Model file for the job. Use its own axes, mm. Give positions to 0.01 mm unless a question says otherwise; leave off trailing zeros. Loops run counter-clockwise (first coordinate to the right, second up) from the corner with the lowest first, then second, coordinate; pieces in that order, holes last. Notation, with made-up numbers: M 83,-15 L 111,-15 A13 ccw 111,8 Z; hole C -8.75,58 d5. An arc over 180 degrees is marked long. Answer in a Markdown table with one row per item.
```python
from build123d import *
from OCP.BRepFilletAPI import BRepFilletAPI_MakeChamfer

# Parameters (mm, degrees)
BOSS_EXTRUDE1_DEPTH = 3
SKETCH2_R           = 2.5
BOSS_EXTRUDE2_DEPTH = 19
LPATTERN1_COUNT     = 2
LPATTERN1_PITCH     = 40
CHAMFER3_SIZE       = 1
CHAMFER3_SIZE2      = 0.624869352
FILLET1_R           = 10
SKETCH_1_R          = 2
CUT_EXTRUDE_1_DEPTH = 49.039445083


with BuildPart() as part:
    # Sketch1 → Boss-Extrude1 (new body)
    with BuildSketch(Plane(origin=(0, 0, 0), x_dir=(1, 0, 0), z_dir=(0, 1, 0))):
        with BuildLine():
            Line((-35, 17.5), (35, 17.5))
            ThreePointArc((35, 17.5), (38.535533906, 16.035533906), (40, 12.5))
            Line((40, 12.5), (40, -17.5))
            Line((40, -17.5), (-40, -17.5))
            Line((-40, -17.5), (-40, 12.5))
            ThreePointArc((-40, 12.5), (-38.535533906, 16.035533906), (-35, 17.5))
        make_face()
    extrude(amount=BOSS_EXTRUDE1_DEPTH)

    # Sketch2 → Boss-Extrude2 (add)
    with BuildSketch(Plane(origin=(40, 0, 0), x_dir=(0, 0, -1), z_dir=(1, 0, 0))):
        with BuildLine():
            Line((-21.372983346, 0), (-17.5, 0))
            Line((-17.5, 0), (-17.5, 3))
            ThreePointArc((-17.5, 3), (-23.822473089, 7.16227766), (-21.372983346, 0))
        make_face()
        with Locations((-21.372983346, 4)):
            Circle(SKETCH2_R, mode=Mode.SUBTRACT)
    boss_extrude2 = extrude(amount=-BOSS_EXTRUDE2_DEPTH)

    # LPattern1: Boss-Extrude2 ×2
    with Locations(*[(-i * LPATTERN1_PITCH, 0, 0) for i in range(1, LPATTERN1_COUNT)]):
        add(boss_extrude2)

    # Chamfer3: one chamfer whose edges measure the first distance from different faces: ONE call of the kernel's chamfer builder (chamfer() names one face for all edges)
    chamfer3_edges_1 = [part.edges().sort_by_distance(p)[0] for p in [
        (-29.5, 3, 17.5),
    ]]
    chamfer3_side_1 = [part.faces().sort_by_distance(p)[0] for p in [
        (-29.5, 1.5, 17.5),
    ]]
    chamfer3_edges_2 = [part.edges().sort_by_distance(p)[0] for p in [
        (10.5, 3, 17.5),
    ]]
    chamfer3_side_2 = [part.faces().sort_by_distance(p)[0] for p in [
        (10.5, 1.5, 17.5),
    ]]
    chamfer3 = BRepFilletAPI_MakeChamfer(part.part.solid().wrapped)
    for e in chamfer3_edges_1:
        chamfer3.Add(CHAMFER3_SIZE, CHAMFER3_SIZE2, e.wrapped, chamfer3_side_1[0].wrapped)  # the first distance lies on this face
    for e in chamfer3_edges_2:
        chamfer3.Add(CHAMFER3_SIZE, CHAMFER3_SIZE2, e.wrapped, chamfer3_side_2[0].wrapped)  # the first distance lies on this face
    add(Compound.cast(chamfer3.Shape()), mode=Mode.REPLACE)

    # Fillet1
    # the kernel refuses this fillet: 10 mm, written as the material it takes off along each edge
    with BuildSketch(Plane(origin=(21, 2, 17.5), x_dir=(0, 0.8480480961564257, -0.5299192642332051), z_dir=(-1, 0, 0))) as fillet1_piece_1:
        with BuildLine():
            CenterArc((2.784251212, 10), FILLET1_R, 243.382335319, 26.617664681)
            Line((-1.696096192, 1.059838528), (0, 0))
            Line((0, 0), (2.784251212, 0))
        make_face()
    extrude(amount=21, mode=Mode.SUBTRACT)
    with BuildSketch(Plane(origin=(-19, 2, 17.5), x_dir=(0, 0.8480480961564257, -0.5299192642332051), z_dir=(-1, 0, 0))) as fillet1_piece_2:
        with BuildLine():
            CenterArc((2.784251212, 10), FILLET1_R, 243.382335319, 26.617664681)
            Line((-1.696096192, 1.059838528), (0, 0))
            Line((0, 0), (2.784251212, 0))
        make_face()
    extrude(amount=27.96062803, mode=Mode.SUBTRACT)

    # 스케치1 → 컷-돌출1 (cut, through all)
    with BuildSketch(Plane.XZ):
        with Locations(Location((-25, 7.372983346, 0), (0, 0, 270))):
            Circle(SKETCH_1_R)
        with Locations(Location((-25, -4.627016654, 0), (0, 0, 270))):
            Circle(SKETCH_1_R)
        with Locations(Location((25, 7.372983346, 0), (0, 0, 270))):
            Circle(SKETCH_1_R)
        with Locations(Location((25, -4.627016654, 0), (0, 0, 270))):
            Circle(SKETCH_1_R)
    extrude(amount=-CUT_EXTRUDE_1_DEPTH, mode=Mode.SUBTRACT)


solid = part.part
```
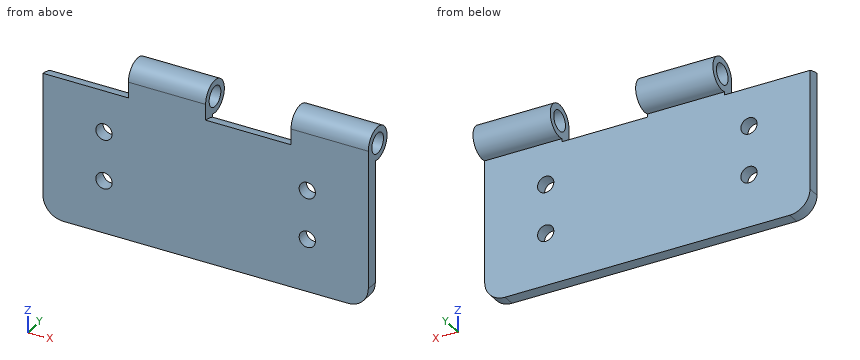
Q1. Probe probe 1 along Z at (x, y) = (-4, 3.75); probe 2 along Y at (x, z) = (17, 6.5); probe 3 along X at (y, z) = (1, 17.5). List the from-to ranges inside material, lowest first.
Reported:
| item | result |
|---|---|
| probe 1 | 17.38 to 18.89, 23.86 to 25.37 |
| probe 2 | 0 to 3 |
| probe 3 | -19 to 0, 21 to 40 |
Q2. Saw through at C-C (x = -25). Give the cut face in (y, z), and give its area (3 significant figures).
Reported:
| item | result |
|---|---|
| outline | M 0,-17.5 L 3,-17.5 L 3,-6.63 L 0,-6.63 Z; M 0,-2.63 L 3,-2.63 L 3,5.37 L 0,5.37 Z; M 0,9.37 L 3,9.37 L 3,16.74 A10 ccw 0,17.5 Z |
| area | 80.1 mm² |
Q3. Saw through at A-A (x = 25). Give the cut face in (y, z).
Reported:
| item | result |
|---|---|
| outline | M 0,-17.5 L 3,-17.5 L 3,-6.63 L 0,-6.63 Z; M 0,-2.63 L 3,-2.63 L 3,5.37 L 0,5.37 Z; M 0,9.37 L 3,9.37 L 3,17.5 A4 ccw long 0,21.37 Z; hole C 4,21.37 d5 |
Q4. Saw through at B-B (y = 4). Give the cut face in (x, z), and give its area (3 significant figures).
Reported:
| item | result |
|---|---|
| outline | M -19,17.37 L 0,17.37 L 0,18.87 L -19,18.87 Z; M -19,23.87 L 0,23.87 L 0,25.37 L -19,25.37 Z; M 21,17.37 L 40,17.37 L 40,18.87 L 21,18.87 Z; M 21,23.87 L 40,23.87 L 40,25.37 L 21,25.37 Z |
| area | 114 mm² |
Q5. Drop flat-ended pins along their axis: pin 1 (6 mm diameter, centred on x = 23.5, z = -2.5, fed in from +Y); pin 2 (3 mm diameter, centred on x = -3.5, y = 1.5, fed in from +Z); pin 3 (8 mm diameter, centred on x = 20, z = 18.5, fed in from +Y); pin 4 (4 mm diameter, centred on y = 2.5, z = 22, fed in from -X). Give the stop position or say it passes through.
Reported:
| item | result |
|---|---|
| pin 1 | y = 3 |
| pin 2 | z = 25.25 |
| pin 3 | y = 8 |
| pin 4 | x = -19 |
Q6. Saw through at D-D (x = -16). Give the cut face in (y, z), and give its area (3 significant figures).
Reported:
| item | result |
|---|---|
| outline | M 0,-17.5 L 3,-17.5 L 3,17.5 A4 ccw long 0,21.37 Z; hole C 4,21.37 d5 |
| area | 139 mm² |
